```python
from build123d import *

# Parameters (mm, degrees)
F0_R     = 4
F0_R_2   = 1
F1_DEPTH = 5


with BuildPart() as f1:
    # F0 (on Front) → F1 (new body)
    with BuildSketch(Plane.XZ):
        Polygon((0, 67), (0, 0), (25.5, 0), (25.5, 67), (20.5, 72), (5, 72), align=None)
        with Locations((12.75, 22.5)):
            Circle(F0_R, mode=Mode.SUBTRACT)
        with Locations((10.25, 63.2)):
            Circle(F0_R_2, mode=Mode.SUBTRACT)
        with Locations((12.75, 50)):
            Circle(F0_R_2, mode=Mode.SUBTRACT)
        with Locations((15.25, 63.2)):
            Circle(F0_R_2, mode=Mode.SUBTRACT)
    extrude(amount=F1_DEPTH)


solid = f1.part
```
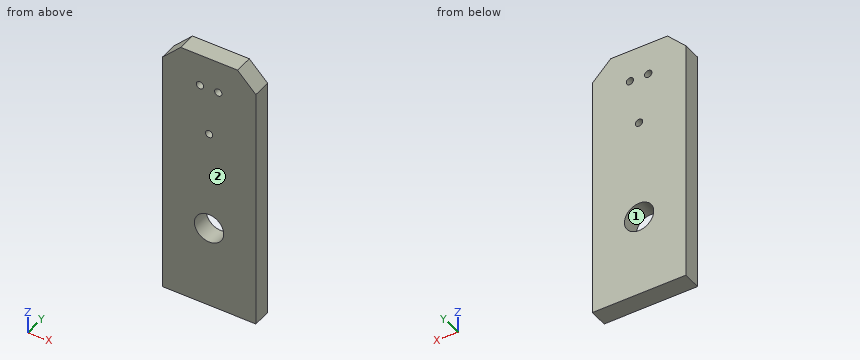
Verification items for the finished model (mm, model axes). Face numbers are marked on the shaded views. Coordinates: 2 decimals unless noted, no trailing zeros. Order: outer loops, then holes, each group sorted by start corner. A loop starts at its lowest first (then second) coordinate and runs counter-clockwise, first axis right, second up. Notation, with made-up numbers: (20.5, 19) -> (58.5, 19) arc R20 cw to (58.5, 27) -> close; hole circle Ø10 at (51, 0). An arc over 180 degrees is marked (long way). Answer as CSV lines item,"result". Start each with the question number.
1) Cross-section at B-B, the plane y = -1.75. Record the boundary of the cut face in (x, z), then the cut area to 3 significant figures.
2) Cross-section at A-A, the plane z = 22.5. Record the boundary of the cut face in (x, y).
3) Cross-section at C-C, the plane x = 13. Record the boundary of the cut face in (y, z).
4) Cross-section at D-D, the plane x = 10.25. Record the boundary of the cut face in (y, z).
5) Release check for a two-part mould opening along X. For the marked faces 1 and 2 record: released by +X, released by -X, zero draft, split by the parting line, or undercut.
6) Material ranges on L1, parallel to Z at x = 12.75, y = -3.7; L2, parallel to X at y = -1.5, z = 62.5; L3, parallel to Z at x = 10.5, y = -1.75, recorded low to high. Write a range as [from, to].
Conclusion:
1,outline,"(0, 0) -> (25.5, 0) -> (25.5, 67) -> (20.5, 72) -> (5, 72) -> (0, 67) -> close; hole circle Ø8 at (12.75, 22.5); hole circle Ø2 at (10.25, 63.2); hole circle Ø2 at (12.75, 50); hole circle Ø2 at (15.25, 63.2)"
1,area,"1,750 mm²"
2,outline,"(0, -5) -> (8.75, -5) -> (8.75, 0) -> (0, 0) -> close; (16.75, -5) -> (25.5, -5) -> (25.5, 0) -> (16.75, 0) -> close"
3,outline,"(-5, 0) -> (0, 0) -> (0, 18.51) -> (-5, 18.51) -> close; (-5, 26.49) -> (0, 26.49) -> (0, 49.03) -> (-5, 49.03) -> close; (-5, 50.97) -> (0, 50.97) -> (0, 72) -> (-5, 72) -> close"
4,outline,"(-5, 0) -> (0, 0) -> (0, 19.38) -> (-5, 19.38) -> close; (-5, 25.62) -> (0, 25.62) -> (0, 62.2) -> (-5, 62.2) -> close; (-5, 64.2) -> (0, 64.2) -> (0, 72) -> (-5, 72) -> close"
5,face 1,"undercut"
5,face 2,"zero draft"
6,L1,"z = [0, 18.5], [26.5, 49], [51, 72]"
6,L2,"x = [0, 9.54], [10.96, 14.54], [15.96, 25.5]"
6,L3,"z = [0, 19.19], [25.81, 62.23], [64.17, 72]"
